Here's how the part is built. I have some questions about the finished solid (model axes, mm). Face numbers are marked on the shaded views. A direction names the side the tool comes from. Coordinates: 2 decimals unless noted, no trailing zeros. Loops run counter-clockwise (first coordinate to the right, second up) from the corner with the lowest first, then second, coordinate; pieces in that order, holes last. Notation, with made-up numbers: M 63,33.5 L 90,33.5 A22 cw 90,44.5 Z; hole C -35,81.5 d10. An arc over 180 degrees is marked long. Use one line per item in the form item = value. Start each with the question number.
(1) Imagine slicing it at D-D, the plane y = 8.5. Please give me the cut outline in (x, z).
(2) Please list where these lines run through material, in increasing order: L1, parallel to X at y = 0, z = 1.3; L2, parallel to Y at x = 0, z = 1.5; L3, parallel to Y at x = 0, z = 11.
(3) Thinking about a two-plate mould opening in Y: for the marked faces 4, 5 and 6, which applies, +Y half, -Y half, draft (parallel to the pull), parting line (faces both ways), or undercut?
(4) Imagine slicing it at C-C, the plane z = 26.5. Please give me the cut outline in (x, y).
(5) Imagine slicing it at A-A, the plane z = 15. Please give me the cut outline in (x, y), and give its area (3 significant figures).
(6) Imagine slicing it at B-B, the plane x = 0. Please give me the cut outline in (y, z), and give its area (3 significant figures).
(7) Will these pins go through, and if not, where does the flat tip stop? P1, Ø2, axis at x = -14.5, y = -16, coming from the -Z side; P2, Ø9, axis at x = -52.5, z = 18, coming from the +Y side; P3, Ø10, axis at y = 17.5, z = 13.5, coming from the +X side; P4, Ø2.5, axis at x = -17, y = 0, coming from the +Z side.
(8) On a 3-axis mill with a long thin cutter (end or side, diameter ignored), from which of +Z, -Z, +X, -X, +Y, -Y can I reach the whole of each face in a straight line? I mean the marked faces 1, 2 and 3. Say none if no direction works.
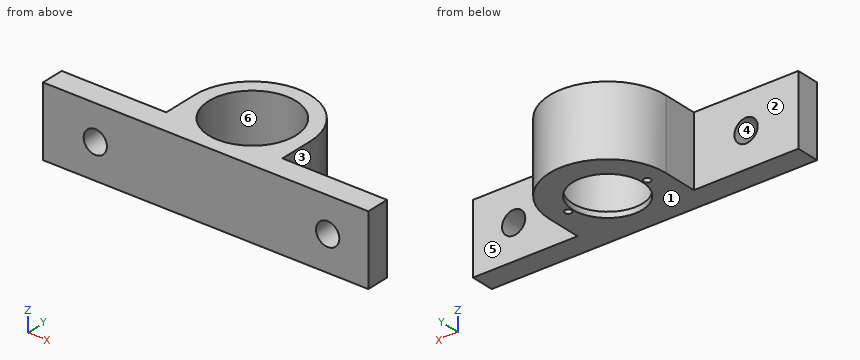
Autodesk Fusion 360 part; units mm, degrees
sketch "Sketch1" plane through (0, 0, 0) normal (0, 0, 1) x (1, 0, 0)
  circle A0 centre (0, 0) radius 18.75
  line L0 (20, -15) -> (20, -25)
  line L1 (20, -25) -> (-20, -25)
  line L2 (-20, -25) -> (-20, -15)
  line L3 (0, -25) -> (50, -25)
  line L4 (50, -25) -> (-50, -25)
  line L5 (-50, -25) -> (-50, -15)
  line L6 (50, -15) -> (50, -25)
  line L7 (-25, 0) -> (-25, -15)
  line L8 (25, 0) -> (25, -15)
  line L9 (-20, -15) -> (-11.25, -15)
  line L10 (11.25, -15) -> (20, -15)
  arc A1 (20, -15) -> (-20, -15) centre (0, 0) ccw
  line L11 (-20, -15) -> (-11.25, -15)
  line L12 (11.25, -15) -> (20, -15)
  line L13 (-50, -15) -> (-11.25, -15)
  line L14 (11.25, -15) -> (50, -15)
  dimension "d1" = 37.5
extrude "Extrude1" add sketch "Sketch1" along normal blind 30 contours A0 L9 L10 A1 L11 L12 L13 L14 | A0 L0 L1 L2 L3 L4 L9 L10 L11 L12 L13 L14 | L7 A1 L13 | L2 L4 L5 L13 | L0 L3 L4 L6 L14 | L8 A1 L14
sketch "Sketch2" plane through (0, 0, 0) normal (0, 0, -1) x (1, 0, 0)
  circle A0 centre (0, 0) radius 18.75
  line L0 (-25, 15) -> (-25, 0)
  arc A1 (-25, 0) -> (25, 0) centre (0, 0) ccw
  line L1 (25, 0) -> (25, 15)
  line L2 (25, 15) -> (50, 15)
  line L3 (50, 15) -> (50, 25)
  line L4 (50, 25) -> (-50, 25)
  line L5 (-50, 25) -> (-50, 15)
  line L6 (-50, 15) -> (-25, 15)
  circle A2 centre (0, 0) radius 15
  line L7 (0, 0) -> (18.75, 0)
  line L8 (18.75, 0) -> (17, 0)
  circle A3 centre (17, 0) radius 1.2
  line L9 (0, 0) -> (0, -15)
  circle A4 centre (-17, 0) radius 1.2
  circle A5 centre (-17, 0) radius 1.5
  circle A6 centre (17, 0) radius 1.5
  dimension "d4" = 30
  dimension "d7" = 2.4
  dimension "d24" = 3
  dimension "d25" = 3
extrude "Extrude3" add sketch "Sketch2" against normal blind 2.4 contours A0 | L7 L8 A3 A6 | L7 L8 A3 A6 | A5
sketch "Sketch3" plane through (0, -15, 0) normal (0, 1, 0) x (-1, 0, 0)
  line L0 (-50, 0) -> (-25, 0)
  line L1 (-25, 0) -> (-25, 30)
  line L2 (-25, 30) -> (-50, 30)
  line L3 (-50, 30) -> (-50, 0)
  line L4 (-50, 30) -> (-37.5, 30)
  line L5 (-37.5, 0) -> (-37.5, 30)
  circle A0 centre (-37.5, 15) radius 6
  line L6 (-50, 30) -> (0, 30)
  line L7 (0, 30) -> (0, 0)
  circle A1 centre (37.5, 15) radius 6
  dimension "d10" = 12
extrude "Extrude5" add 1 faces at (50, -18.3333, 10) along direction (1, 0, 0) blind 20
extrude "Extrude6" add 1 faces at (-50, -21.6667, 10) along direction (-1, 0, 0) blind 20
sketch "Sketch4" plane through (0, -15, 0) normal (0, 1, 0) x (-1, 0, 0)
  line L0 (25, 0) -> (70, 0)
  line L1 (70, 0) -> (70, 30)
  line L2 (70, 30) -> (25, 30)
  line L3 (25, 30) -> (25, 0)
  line L4 (70, 0) -> (47.5, 0)
  circle A0 centre (47.5, 15) radius 5
  circle A1 centre (-52.5, 15) radius 5
  line L5 (47.5, 0) -> (47.5, 10)
  line L6 (47.5, 20) -> (47.5, 30)
  dimension "d19" = 10
  dimension "d20" = 100
  dimension "d21" = 10
extrude "Extrude7" cut sketch "Sketch4" against normal blind 24 contours A0 | A1
extrude "Extrude8" cut sketch "Sketch2" against normal blind 26 contours A5
extrude "Extrude9" cut sketch "Sketch2" against normal blind 40 contours L7 L8 A3 A6 | L7 L8 A3 A6
Answer:
q1.outline = M -23.51,0 L -12.36,0 L -12.36,2.4 L -16.71,2.4 L -16.71,30 L -23.51,30 Z; M 12.36,0 L 23.51,0 L 23.51,30 L 16.71,30 L 16.71,2.4 L 12.36,2.4 Z
q2.L1 = -25 to -18.5, -15.5 to -15, 15 to 15.5, 18.5 to 25
q2.L2 = -25 to -15, 15 to 25
q2.L3 = -25 to -18.75, 18.75 to 25
q3.face_4 = draft
q3.face_5 = +Y half
q3.face_6 = undercut
q4.outline = M -70,-25 L 70,-25 L 70,-15 L 25,-15 L 25,0 A25 ccw -25,0 L -25,-15 L -70,-15 Z; hole C 0,0 d37.5
q5.outline = M -70,-25 L -52.5,-25 L -52.5,-15 L -70,-15 Z; M -42.5,-25 L 47.5,-25 L 47.5,-15 L 25,-15 L 25,0 A25 ccw -25,0 L -25,-15 L -42.5,-15 Z; M 57.5,-25 L 70,-25 L 70,-15 L 57.5,-15 Z; hole C 0,0 d37.5
q5.area = 1,830 mm²
q6.outline = M -25,0 L -15,0 L -15,2.4 L -18.75,2.4 L -18.75,30 L -25,30 Z; M 15,0 L 25,0 L 25,30 L 18.75,30 L 18.75,2.4 L 15,2.4 Z
q6.area = 393 mm²
q7.P1 = 0
q7.P2 = -15
q7.P3 = 21.65
q7.P4 = through
q8.face_1 = -Z, +X, -X, +Y, -Y
q8.face_2 = +Z, -Z, -X, +Y
q8.face_3 = +Z, -Z, +X, +Y
